For this review, use the dimensioned drawing (mm, ordinates from the lowest corner) and the shaded views. Coordinates: 2 decimals unless noted, no trailing zeros. Write each loop counter-clockwise with the first axis right and the second up, starting at its lowest first coordinate (ties: lowest second). Pieces come first, ordered by that corner, then holes. Notation, with made-up numbers: M 87.5,32 L 118.5,32 A26 cw 118.5,49 Z; hole C 38.5,11.5 d5. An arc over 180 degrees is marked long. Return JSON: item names as keys, results as strings.
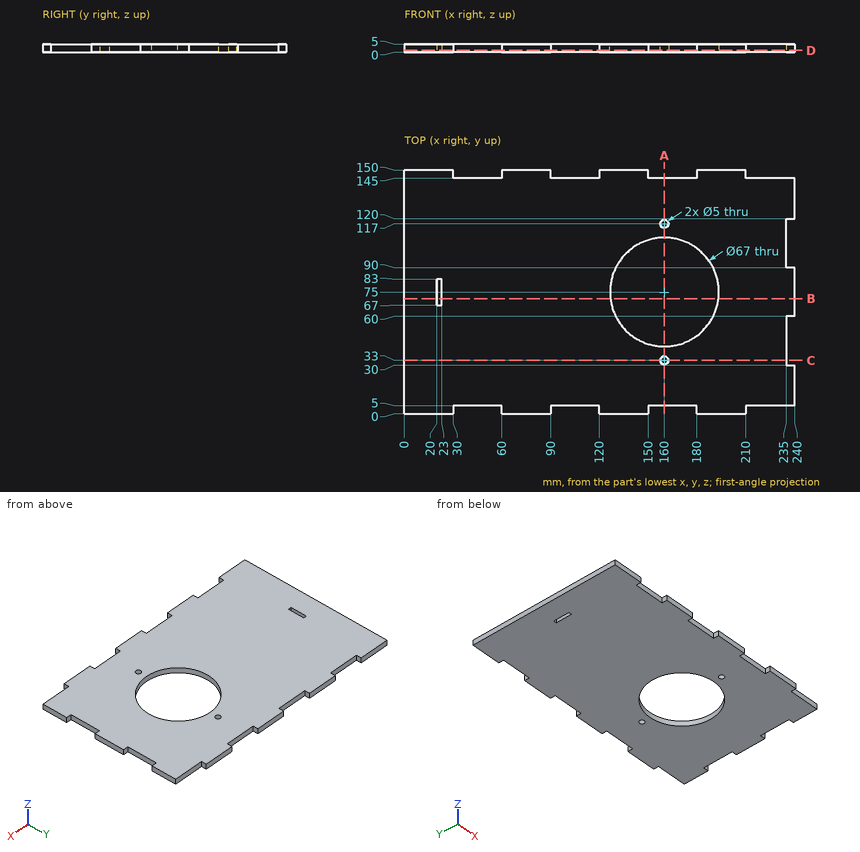
1. Clearance check with flat-ended pins moving along their axes: pin 1 Ø2.5 at (x, z) = (50, 2) entering from +Y; pin 2 Ø2.5 at (y, z) = (2, 3) entering from +X; pin 3 Ø2.5 at (x, z) = (51.5, 2) entering from -Y. State where each tip first meets the part, or that it passes through.
Checks:
{"pin 1": "y = 145", "pin 2": "x = 210", "pin 3": "y = 5"}
2. Wall thickness on L1, parallel to Y at x = 160, z = 2.5; L2, parallel to X at y = 33, z = 1.35; L3, parallel to Y at x = 187, z = 1.85: over which ranges is each line inside the solid? List them lowest first. Write a range as from..to.
Checks:
{"L1": "5..30.5, 35.5..41.5, 108.5..114.5, 119.5..145", "L2": "0..157.5, 162.5..235", "L3": "0..55.17, 94.83..150"}
3. We need section D-D (z = 1.05). Give the number of separate pieces and of enclosed holes in the cut face, plus the area to 3 significant figures.
Checks:
{"separate pieces": "1", "enclosed holes": "4", "area": "30,900 mm2"}
4. We need section A-A (x = 160). State the section outline as (y, z) points.
Checks:
{"outline": "M 5,0 L 30.5,0 L 30.5,5 L 5,5 Z; M 35.5,0 L 41.5,0 L 41.5,5 L 35.5,5 Z; M 108.5,0 L 114.5,0 L 114.5,5 L 108.5,5 Z; M 119.5,0 L 145,0 L 145,5 L 119.5,5 Z"}
5. We need section C-C (y = 33). State the section outline as (x, z) points.
Checks:
{"outline": "M 0,0 L 157.5,0 L 157.5,5 L 0,5 Z; M 162.5,0 L 235,0 L 235,5 L 162.5,5 Z"}
6. We need section B-B (y = 71). State the section outline as (x, z) points.
Checks:
{"outline": "M 0,0 L 20,0 L 20,5 L 0,5 Z; M 23,0 L 126.74,0 L 126.74,5 L 23,5 Z; M 193.26,0 L 240,0 L 240,5 L 193.26,5 Z"}
